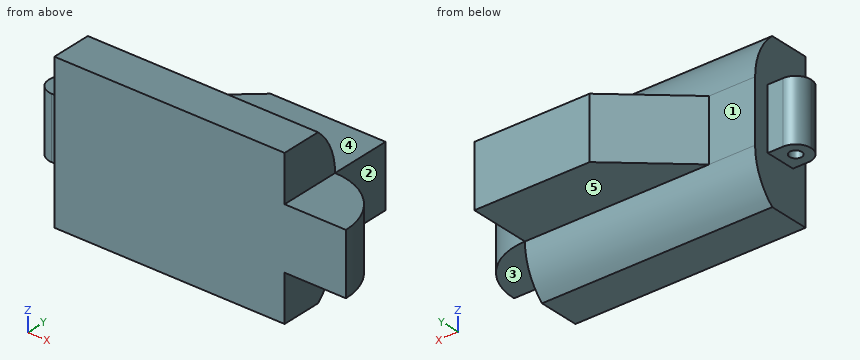
from build123d import *

# Parameters (mm, degrees)
SKETCH1_W           = 95.25
SKETCH1_H           = 63.5
BOSS_EXTRUDE1_DEPTH = 25.4
SKETCH2_W           = 76.2
SKETCH2_H           = 25.4
BOSS_EXTRUDE2_DEPTH = 25.4
CUT_EXTRUDE1_DEPTH  = 25.4
SKETCH4_W           = 25.4
SKETCH4_H           = 25.4
BOSS_EXTRUDE3_DEPTH = 25.4
CUT_EXTRUDE2_DEPTH  = 25.4
CUT_EXTRUDE3_DEPTH  = 95.25
SKETCH_1648_W       = 25.4
SKETCH_1648_H       = 12.7
BOSS_EXTRUDE4_DEPTH = 12.7
CUT_EXTRUDE4_DEPTH  = 25.4
SKETCH10_R          = 2.54
CUT_EXTRUDE5_DEPTH  = 25.4
SCALE1_SCALE        = 0.5


with BuildPart() as part:
    # Sketch1 → Boss-Extrude1 (new body)
    with BuildSketch(Plane(origin=(0, 0, 0), x_dir=(1, 0, 0), z_dir=(0, 1, 0))):
        Rectangle(SKETCH1_W, SKETCH1_H)
    extrude(amount=BOSS_EXTRUDE1_DEPTH)

    # Sketch2 → Boss-Extrude2 (add)
    with BuildSketch(Plane(origin=(0, 25.4, 0), x_dir=(1, 0, 0), z_dir=(0, 1, 0))):
        with Locations((9.525, 0)):
            Rectangle(SKETCH2_W, SKETCH2_H)
    extrude(amount=BOSS_EXTRUDE2_DEPTH)

    # Sketch3 → Cut-Extrude1 (cut)
    with BuildSketch(Plane.XY.offset(12.7)):
        Polygon((-28.575, 50.8), (-28.575, 25.4), (0, 50.8), align=None)
    extrude(amount=-CUT_EXTRUDE1_DEPTH, mode=Mode.SUBTRACT)

    # Sketch4 → Boss-Extrude3 (add)
    with BuildSketch(Plane(origin=(47.625, 0, 0), x_dir=(0, 0, -1), z_dir=(1, 0, 0))):
        with Locations((0, 12.7)):
            Rectangle(SKETCH4_W, SKETCH4_H)
    extrude(amount=BOSS_EXTRUDE3_DEPTH)

    # Sketch5 → Cut-Extrude2 (cut)
    with BuildSketch(Plane(origin=(0, 0, -12.7), x_dir=(-1, 0, 0), z_dir=(0, 0, -1))):
        with BuildLine():
            ThreePointArc((-47.625, 25.4), (-65.585512242, 17.960512242), (-73.025, 0))
            Line((-73.025, 0), (-73.025, 25.4))
            Line((-73.025, 25.4), (-47.625, 25.4))
        make_face()
    extrude(amount=-CUT_EXTRUDE2_DEPTH, mode=Mode.SUBTRACT)

    # Sketch7 → Cut-Extrude3 (cut)
    with BuildSketch(Plane(origin=(47.625, 0, 0), x_dir=(0, 0, -1), z_dir=(1, 0, 0))):
        with BuildLine():
            Line((-31.75, 16.800520825), (-31.75, 25.4))
            Line((-31.75, 25.4), (-12.7, 25.4))
            ThreePointArc((-12.7, 25.4), (-23.150520825, 23.150520825), (-31.75, 16.800520825))
        make_face()
        with BuildLine():
            Line((12.7, 25.4), (31.75, 25.4))
            Line((31.75, 25.4), (31.75, 16.800520825))
            ThreePointArc((31.75, 16.800520825), (23.150520825, 23.150520825), (12.7, 25.4))
        make_face()
    extrude(amount=-CUT_EXTRUDE3_DEPTH, mode=Mode.SUBTRACT)

    # Sketch 1648 → Boss-Extrude4 (add)
    with BuildSketch(Plane.ZY.offset(47.625)):
        with Locations((0, 12.7)):
            Rectangle(SKETCH_1648_W, SKETCH_1648_H)
    extrude(amount=BOSS_EXTRUDE4_DEPTH)

    # Sketch9 → Cut-Extrude4 (cut)
    with BuildSketch(Plane.XY.offset(12.7)):
        with BuildLine():
            ThreePointArc((-53.975, 6.35), (-58.465128061, 8.209871939), (-60.325, 12.7))
            Line((-60.325, 12.7), (-60.325, 6.35))
            Line((-60.325, 6.35), (-53.975, 6.35))
        make_face()
        with BuildLine():
            Line((-60.325, 19.05), (-60.325, 12.7))
            ThreePointArc((-60.325, 12.7), (-58.465128061, 17.190128061), (-53.975, 19.05))
            Line((-53.975, 19.05), (-60.325, 19.05))
        make_face()
    extrude(amount=-CUT_EXTRUDE4_DEPTH, mode=Mode.SUBTRACT)

    # Sketch10 → Cut-Extrude5 (cut)
    with BuildSketch(Plane.XY.offset(12.7)):
        with Locations((-53.975, 12.7)):
            Circle(SKETCH10_R)
    extrude(amount=-CUT_EXTRUDE5_DEPTH, mode=Mode.SUBTRACT)


with BuildPart() as part_1:
    # Scale1: scaled about (6.140340788, 16.964715806, 0)
    add(part.part.scale(SCALE1_SCALE).moved(Location((3.070170394, 8.482357903, 0))))


solid = part_1.part
The listing builds one solid part. Answer for the finished solid, in the listing's coordinates (mm). Face numbers are marked on the shaded views. A direction names the side the tool comes from. Coordinates: 2 decimals unless noted, no trailing zeros. Write each loop counter-clockwise with the first axis right and the second up, starting at its lowest first coordinate (ties: lowest second). Pieces come first, ordered by that corner, then holes. Notation, with made-up numbers: (72.5, -29) - (116.5, -29) arc R25 ccw to (116.5, -9) - close; hole circle Ø5 at (39.25, 75). An arc over 180 degrees is marked (long way). Answer as CSV lines item,"result".
1. Straight lines are drawn through the part: line 1 (X direction, y = 19.25, z = -12); line 2 (Z direction, x = 17, y = 25.5); line 3 (X direction, y = 14.5, z = 0). For each, find the intervals that lie inside material, in ascending order. Write a range as [from, to].
Computed values:
line 1,"x = [-20.74, 26.88]"
line 2,"z = [-6.35, 6.35]"
line 3,"x = [-27.07, -25.14], [-22.69, 38.07]"
2. Find section C-C (y = 20). Give the vertices of the cut face in (x, z).
Computed values:
outline,"(-20.74, -11.7) - (26.88, -11.7) - (26.88, -6.35) - (32.23, -6.35) - (32.23, 6.35) - (26.88, 6.35) - (26.88, 11.7) - (-20.74, 11.7) - close"
3. Find section B-B (x = 25.5). Give the vertices of the cut face in (y, z) (3 decimals).
Computed values:
outline,"(8.482, -15.875) - (16.883, -15.875) arc R12.7 ccw to (21.182, -6.35) - (33.882, -6.35) - (33.882, 6.35) - (21.182, 6.35) arc R12.7 ccw to (16.883, 15.875) - (8.482, 15.875) - close"
4. A tool of negligible diameter and unlimited length cuts with its end or side. For the marked faces 1, 2, 3, 4 and 5, from which of +Z, -Z, +X, -X, +Y, -Y can it reach the whole face along a straight path? Write none if from no direction.
Computed values:
face 1,"+Z, -Z, -X, +Y"
face 2,"+Z, -Z, +X, +Y"
face 3,"-Z, +X, +Y, -Y"
face 4,"+Z, +X, -X, +Y"
face 5,"-Z, +X, -X, +Y"
5. Find section D-D (x = -16.5). Give the vertices of the cut face in (y, z) (3 decimals), plus the area to 3 significant figures.
Computed values:
outline,"(8.482, -15.875) - (16.883, -15.875) arc R12.7 ccw to (21.182, -6.35) - (21.182, 6.35) arc R12.7 ccw to (16.883, 15.875) - (8.482, 15.875) - close"
area,"378 mm²"
6. Given P1, Ø10, axis at y = 30.5, z = 0.5, coming from the +X side; P2, Ø3, axis at y = 29, z = 4.5, coming from the -X side; P3, Ø10, axis at y = 21.5, z = -7, coming from the +X side, each flat-ended and moving along its own axis, determine where each tip first touches the part or whether it passes through.
Computed values:
P1,"stops at x = 26.88"
P2,"stops at x = -4.11"
P3,"stops at x = 36.7"
7. Find section A-A (z = 1). Give the vertices of the cut face in (x, y) (3 decimals).
Computed values:
outline,"(-23.917, 11.657) - (-20.742, 11.657) - (-20.742, 8.482) - (39.583, 8.482) arc R12.7 ccw to (26.883, 21.182) - (26.883, 33.882) - (3.07, 33.882) - (-11.217, 21.182) - (-20.742, 21.182) - (-20.742, 18.007) - (-23.917, 18.007) arc R3.175 ccw to start; hole circle Ø2.54 at (-23.917, 14.832)"
